from build123d import *

# Parameters (mm, degrees)
CYLINDER004_R          = 2
CYLINDER004_DEPTH      = 16
CYLINDER004_ROLL_ANGLE = -90
BOX001_W               = 5
BOX001_H               = 8
BOX001_DEPTH           = 8
CYLINDER006_R          = 2
CYLINDER006_DEPTH      = 30
CYLINDER006_ROLL_ANGLE = -90
CYLINDER003_R          = 10.2
CYLINDER003_DEPTH      = 20
CYLINDER003_ROLL_ANGLE = -90
CYLINDER005_R          = 2
CYLINDER005_DEPTH      = 30
CYLINDER002_R          = 10.2
CYLINDER002_DEPTH      = 28
BOX_W                  = 10
BOX_H                  = 4
BOX_DEPTH              = 10
BOX002_W               = 10
BOX002_H               = 4
BOX002_DEPTH           = 10
CYLINDER001_R          = 14
CYLINDER001_DEPTH      = 16
CYLINDER001_ROLL_ANGLE = -90
CYLINDER_R             = 14
CYLINDER_DEPTH         = 16


with BuildPart() as cylinder004:
    # Cylinder004 → Cylinder004 (new body)
    with BuildSketch(Plane.XY):
        Circle(CYLINDER004_R)
    extrude(amount=CYLINDER004_DEPTH)


with BuildPart() as cylinder004_1:
    # Cylinder004 roll: moved
    add(cylinder004.part.rotate(Axis((0, 0, 0), (1, 0, 0)), CYLINDER004_ROLL_ANGLE))


with BuildPart() as cylinder004_2:
    # Cylinder004 placement: moved
    add(cylinder004_1.part.moved(Location((-25, -8, 0))))


with BuildPart() as cube001:
    # Box001 → Box001 (new body)
    with BuildSketch(Plane(origin=(-24, -4, -4), x_dir=(1, 0, 0), z_dir=(0, 0, 1))):
        with Locations((2.5, 4)):
            Rectangle(BOX001_W, BOX001_H)
    extrude(amount=BOX001_DEPTH)


with BuildPart() as cylinder006:
    # Cylinder006 → Cylinder006 (new body)
    with BuildSketch(Plane.XY):
        Circle(CYLINDER006_R)
    extrude(amount=CYLINDER006_DEPTH)


with BuildPart() as cylinder006_1:
    # Cylinder006 roll: moved
    add(cylinder006.part.rotate(Axis((0, 0, 0), (1, 0, 0)), CYLINDER006_ROLL_ANGLE))


with BuildPart() as cylinder006_2:
    # Cylinder006 placement: moved
    add(cylinder006_1.part.moved(Location((-10, -15, 0))))


with BuildPart() as cylinder003:
    # Cylinder003 → Cylinder003 (new body)
    with BuildSketch(Plane.XY):
        Circle(CYLINDER003_R)
    extrude(amount=CYLINDER003_DEPTH)


with BuildPart() as cylinder003_1:
    # Cylinder003 roll: moved
    add(cylinder003.part.rotate(Axis((0, 0, 0), (1, 0, 0)), CYLINDER003_ROLL_ANGLE))


with BuildPart() as cylinder003_2:
    # Cylinder003 placement: moved
    add(cylinder003_1.part.moved(Location((10, -10, 0))))


with BuildPart() as cylinder005:
    # Cylinder005 → Cylinder005 (new body)
    with BuildSketch(Plane(origin=(10, 0, -15), x_dir=(1, 0, 0), z_dir=(0, 0, 1))):
        Circle(CYLINDER005_R)
    extrude(amount=CYLINDER005_DEPTH)


with BuildPart() as negative_fusion:
    # Cylinder002 → Cylinder002 (new body)
    with BuildSketch(Plane(origin=(-10, 0, -10), x_dir=(1, 0, 0), z_dir=(0, 0, 1))):
        Circle(CYLINDER002_R)
    extrude(amount=CYLINDER002_DEPTH)

    # Fusion001: union Cylinder004, Cube001, Cylinder006, Cylinder003, Cylinder005
    add(cylinder004_2.part)
    add(cube001.part)
    add(cylinder006_2.part)
    add(cylinder003_2.part)
    add(cylinder005.part)


with BuildPart() as cube:
    # Box → Box (new body)
    with BuildSketch(Plane(origin=(-30, -8, -5), x_dir=(1, 0, 0), z_dir=(0, 0, 1))):
        with Locations((5, 2)):
            Rectangle(BOX_W, BOX_H)
    extrude(amount=BOX_DEPTH)


with BuildPart() as cube002:
    # Box002 → Box002 (new body)
    with BuildSketch(Plane(origin=(-30, 4, -5), x_dir=(1, 0, 0), z_dir=(0, 0, 1))):
        with Locations((5, 2)):
            Rectangle(BOX002_W, BOX002_H)
    extrude(amount=BOX002_DEPTH)


with BuildPart() as cylinder001:
    # Cylinder001 → Cylinder001 (new body)
    with BuildSketch(Plane.XY):
        Circle(CYLINDER001_R)
    extrude(amount=CYLINDER001_DEPTH)


with BuildPart() as cylinder001_1:
    # Cylinder001 roll: moved
    add(cylinder001.part.rotate(Axis((0, 0, 0), (1, 0, 0)), CYLINDER001_ROLL_ANGLE))


with BuildPart() as cylinder001_2:
    # Cylinder001 placement: moved
    add(cylinder001_1.part.moved(Location((10, -8, 0))))


with BuildPart() as cut:
    # Cylinder → Cylinder (new body)
    with BuildSketch(Plane(origin=(-10, 0, -8), x_dir=(1, 0, 0), z_dir=(0, 0, 1))):
        Circle(CYLINDER_R)
    extrude(amount=CYLINDER_DEPTH)

    # Fusion: union Cube, Cube002, Cylinder001
    add(cube.part)
    add(cube002.part)
    add(cylinder001_2.part)

    # Cut: cut Negative Fusion
    add(negative_fusion.part, mode=Mode.SUBTRACT)


solid = cut.part
CAD build for the part. Positions are in the model's coordinates, mm. A direction names the side the tool comes from. Round coordinates to 2 decimals unless told otherwise and drop trailing zeros. Loops run counter-clockwise (first coordinate to the right, second up) from the corner with the lowest first, then second, coordinate; pieces in that order, holes last. Notation, with made-up numbers: (-6, 2) - (16, 2) arc R17 cw to (16, 6) - close; hole circle Ø8 at (12, -28.5). An arc over 180 degrees is marked (long way). Put each result on its own line as item: value.
1. Slice it at D-D on y = 1.25. List the corners of the cut face in (x, z), and give its area (3 significant figures).
Geometry check:
outline: (-23.94, -8) - (-20.12, -8) - (-20.12, -4) - (-23.94, -4) - close; (-23.94, 4) - (-20.12, 4) - (-20.12, 8) - (-23.94, 8) - close; (0.12, -9.92) arc R14 ccw to (8.44, -13.91) - (8.44, -10.08) arc R10.2 cw to (0.12, -2.55) - close; (0.12, 2.55) arc R10.2 cw to (8.44, 10.08) - (8.44, 13.91) arc R14 ccw to (0.12, 9.92) - close; (11.56, -13.91) arc R14 ccw to (11.56, 13.91) - (11.56, 10.08) arc R10.2 cw to (11.56, -10.08) - close
area: 240 mm²
2. 3-axis set-ups, long thin cutter, end or side, ignore diameter. For faces 1 (the flat face through (-27, -6, 5)), 2 (the cylindrical face through (8.4, -1.2, -12)), 3 (the flat face through (-27, 6, -5)), 4 (the flat face through (-22, 0, 4)), 5 (the flat face through (-27, 6, 5)): which of +Z, -Z, +X, -X, +Y, -Y reach the whole face in a straight line?
Geometry check:
face 1: +Z, -X, -Y
face 2: +Z, -Z
face 3: -Z, -X, +Y
face 4: -X
face 5: +Z, -X, +Y
3. Slice it at A-A on x = -25. List the corners of the cut face in (y, z).
Geometry check:
outline: (-8, -5) - (-4, -5) - (-4, -2) - (-8, -2) - close; (-8, 2) - (-4, 2) - (-4, 5) - (-8, 5) - close; (4, -5) - (8, -5) - (8, -2) - (4, -2) - close; (4, 2) - (8, 2) - (8, 5) - (4, 5) - close
4. Slice it at B-B on y = 7.25. List the corners of the cut face in (x, z), and give its area (3 significant figures).
Geometry check:
outline: (-30, -5) - (-21.98, -5) - (-21.98, -8) - (-17.17, -8) - (-17.17, 8) - (-21.98, 8) - (-21.98, 5) - (-30, 5) - close; (-2.83, -8) - (-1.49, -8) arc R14 ccw (long way) to (-1.49, 8) - (-2.83, 8) - close; hole circle Ø4 at (-25, 0); hole circle Ø20.4 at (10, 0)
area: 427 mm²
5. Pin check, flat tips, straight feed: P1, Ø3, axis at x = -27, y = -5.5, coming from the +Z side; P2, Ø8, axis at x = 3.5, z = -2, coming from the +Y side; P3, Ø2.5, axis at x = -22.5, y = 0, coming from the -Z side; P4, Ø3, axis at x = -25, z = 0, coming from the +Y side. Stop position of each tip, or through.
Geometry check:
P1: z = 5
P2: y = 10.28
P3: z = -8
P4: through
6. Wall check: line 1 (Z direction, x = -25, y = -7.75); line 2 (X direction, y = 0, z = -4.25); line 3 (Z direction, x = -10, y = 12.95). Give the ranges that are in metal, low to high.
Geometry check:
line 1: -5 to -2, 2 to 5
line 2: -24 to -20.2, 0.2 to 0.73, 19.27 to 23.34
line 3: -8 to -2, 2 to 8
7. Slice it at C-C on z = 0. Give the number of separate pieces and of enclosed holes in the cut face, and give its area (3 significant figures).
Geometry check:
separate pieces: 7
enclosed holes: 0
area: 259 mm²
8. Two-plate mould, pull along Z, no slides. Class faces 6 (the flat face through (-20, 5, -8)), 7 (the flat face through (-22, 0, -4)), 8 (the flat face through (21, -8, 1)), 9 (the cylindrical face through (-27, 6, 0)): released by +Z, released by -Z, zero draft, split by the parting line, or undercut.
Geometry check:
face 6: released by -Z
face 7: undercut
face 8: zero draft
face 9: undercut
